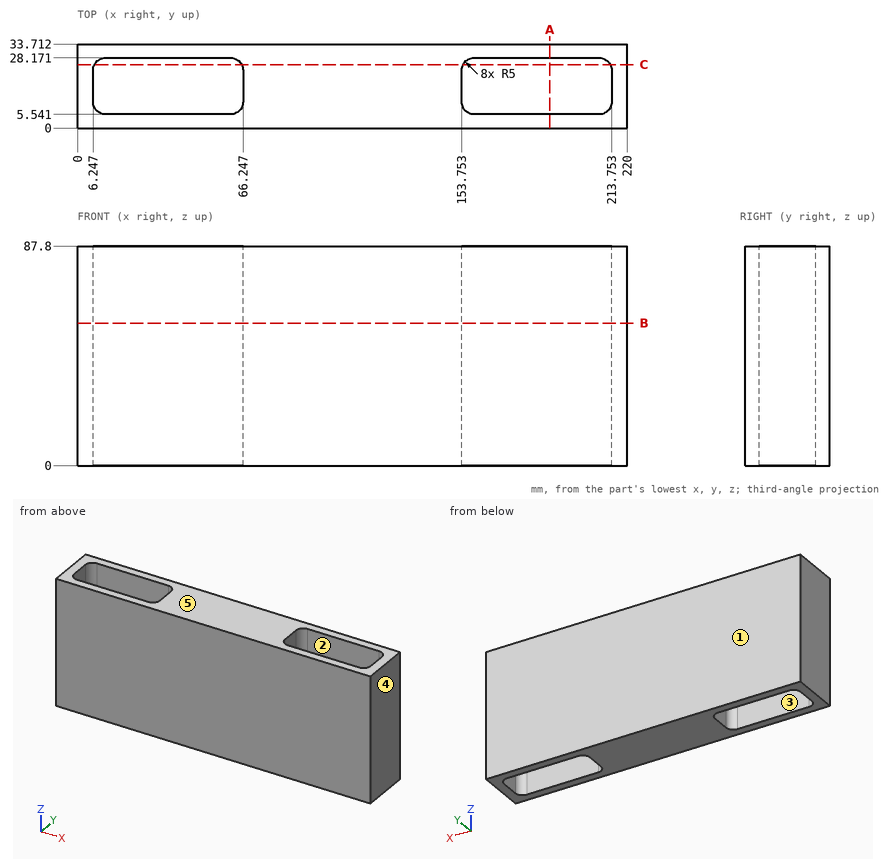
For this review, use the dimensioned drawing (mm, ordinates from the lowest corner) and the shaded views. A direction names the side the tool comes from. Give positions to 0.01 mm unless a question says otherwise; leave off trailing zeros. Order: outer loops, then holes, each group sorted by start corner. A loop starts at its lowest first (then second) coordinate and runs counter-clockwise, first axis right, second up. Notation, with made-up numbers: (23, -31.5) - (39, -31.5) arc R27 cw to (39, 7.5) - close; hole circle Ø5 at (-34, 42.25). An arc over 180 degrees is marked (long way). Write item = value, one per line. Start each with the question number.
Q1. Tool access review of the marked faces 1 and 2: name each direction out of +Z, -Z, +X, -X, +Y, -Y from which nothing blocks a thin tool from reaching the whole face with its end or side.
Q2. We need section B-B on z = 57. State the section outline as (x, y) points.
Q3. We need section C-C on y = 25.5. State the section outline as (x, z) points, plus the area to 3 significant figures.
Q4. Mouldability with a two-part tool opening along X and no side actions: class the marked faces 3, 4 and 5 as released by +X, released by -X, zero draft, split by the parting line, or undercut.
Q5. To check wall thickness, follow L1, parallel to X at y = 11.5, z = 67; L2, parallel to Y at x = 203.5, z = 32; L3, parallel to X at y = 7.5, z = 61.5. State the ranges of each line that lie inside material, in increasing order. Write a range as from..to.
Q6. We need section A-A on x = 189. State the section outline as (y, z) points, plus the area to 3 significant figures.
Working result:
q1.face_1 = +Z, -Z, +X, -X, +Y
q1.face_2 = +Z, -Z
q2.outline = (0, 0) - (220, 0) - (220, 33.71) - (0, 33.71) - close; hole (6.25, 10.54) arc R5 ccw to (11.25, 5.54) - (61.25, 5.54) arc R5 ccw to (66.25, 10.54) - (66.25, 23.17) arc R5 ccw to (61.25, 28.17) - (11.25, 28.17) arc R5 ccw to (6.25, 23.17) - close; hole (153.75, 10.54) arc R5 ccw to (158.75, 5.54) - (208.75, 5.54) arc R5 ccw to (213.75, 10.54) - (213.75, 23.17) arc R5 ccw to (208.75, 28.17) - (158.75, 28.17) arc R5 ccw to (153.75, 23.17) - close
q3.outline = (0, 0) - (6.82, 0) - (6.82, 87.8) - (0, 87.8) - close; (65.67, 0) - (154.33, 0) - (154.33, 87.8) - (65.67, 87.8) - close; (213.18, 0) - (220, 0) - (220, 87.8) - (213.18, 87.8) - close
q3.area = 8,980 mm²
q4.face_3 = undercut
q4.face_4 = released by +X
q4.face_5 = zero draft
q5.L1 = 0..6.25, 66.25..153.75, 213.75..220
q5.L2 = 0..5.54, 28.17..33.71
q5.L3 = 0..7.28, 65.22..154.78, 212.72..220
q6.outline = (0, 0) - (5.54, 0) - (5.54, 87.8) - (0, 87.8) - close; (28.17, 0) - (33.71, 0) - (33.71, 87.8) - (28.17, 87.8) - close
q6.area = 973 mm²
